Verification items for the finished model (mm, model axes). A direction names the side the tool comes from. Give positions to 0.01 mm unless a question says otherwise; leave off trailing zeros. Loops run counter-clockwise (first coordinate to the right, second up) from the corner with the lowest first, then second, coordinate; pieces in that order, holes last. Notation, with made-up numbers: (-11.75, -8) - (19.25, -8) arc R24 ccw to (19.25, 13) - close; hole circle Ø3 at (-36, 34). An arc over 180 degrees is marked (long way). Answer in a Markdown table with one row per item.
```python
from build123d import *

# Parameters (mm, degrees)
EXTRUDE_1_DEPTH             = 43.4
EXTRUDE_2_DEPTH             = 1.8
CUT_EXTRUDE_1_DEPTH         = 43.4
EXTRUDE_3_DEPTH             = 43.4
EXTRUDE_4_DEPTH             = 16.205128205
SKETCH_6_W                  = 45.2
SKETCH_6_H                  = 41
EXTRUDE_5_DEPTH             = 2
SKETCH_7_W                  = 34
SKETCH_7_H                  = 20
EXTRUDE_6_DEPTH             = 8
EXTRUDE_7_DEPTH             = 1.8
HOLE_WIZARD_3_3_3_3_2_D     = 3.3
HOLE_WIZARD_3_3_3_3_2_DEPTH = 10
HOLE_WIZARD_16_0_16_1_D     = 16
HOLE_WIZARD_16_0_16_1_DEPTH = 55
SKETCH_19_R                 = 1.65
CUT_EXTRUDE_6_DEPTH         = 5


with BuildPart() as part:
    # 草图1 → 凸台-拉伸1 (new body)
    with BuildSketch(Plane(origin=(21.7, 0, 0), x_dir=(0, 0, -1), z_dir=(1, 0, 0))):
        Polygon((-18.205128205, 8), (-18.205128205, 49), (-55, 8), align=None)
    extrude(amount=-EXTRUDE_1_DEPTH)

    # 草图2 → 凸台-拉伸2 (add)
    with BuildSketch(Plane.ZY.offset(21.7)):
        Polygon((18.205128205, 8), (18.205128205, 49), (55, 8), align=None)
    extrude(amount=EXTRUDE_2_DEPTH)

    # 草图3 → 切除-拉伸1 (cut)
    with BuildSketch(Plane(origin=(21.7, 0, 0), x_dir=(0, 0, -1), z_dir=(1, 0, 0))):
        Polygon((-18.205128205, 8), (-18.205128205, 47), (-20, 47), (-55, 8), align=None)
    extrude(amount=-CUT_EXTRUDE_1_DEPTH, mode=Mode.SUBTRACT)

    # 草图4 → 凸台-拉伸3 (add)
    with BuildSketch(Plane(origin=(-21.7, 0, 0), x_dir=(0, 0, -1), z_dir=(1, 0, 0))):
        Polygon((-18.205128205, 10), (-18.205128205, 8), (-55, 8), (-53.205128205, 10), align=None)
    extrude(amount=EXTRUDE_3_DEPTH)

    # 草图5 → 凸台-拉伸4 (add)
    with BuildSketch(Plane(origin=(0, 0, 18.205128205), x_dir=(-1, 0, 0), z_dir=(0, 0, -1))):
        Polygon((21.7, 10), (21.7, 47), (-21.7, 47), (-21.7, 49), (23.5, 49), (23.5, 8), (-21.7, 8), (-21.7, 10), align=None)
    extrude(amount=EXTRUDE_4_DEPTH)

    # 草图6 → 凸台-拉伸5 (add)
    with BuildSketch(Plane(origin=(0, 0, 2), x_dir=(-1, 0, 0), z_dir=(0, 0, -1))):
        with Locations((0.9, 28.5)):
            Rectangle(SKETCH_6_W, SKETCH_6_H)
    extrude(amount=EXTRUDE_5_DEPTH)

    # 草图7 → 凸台-拉伸6 (add)
    with BuildSketch(Plane.XZ.offset(-8)):
        with Locations((0, 10)):
            Rectangle(SKETCH_7_W, SKETCH_7_H)
    extrude(amount=EXTRUDE_6_DEPTH)

    # 草图10 → 凸台-拉伸7 (add)
    with BuildSketch(Plane(origin=(21.7, 0, 0), x_dir=(0, 0, -1), z_dir=(1, 0, 0))):
        Polygon((0, 49), (0, 8), (-55, 8), (-18.205128205, 49), align=None)
    extrude(amount=EXTRUDE_7_DEPTH)

    # Ø3.3 (3.3) 直径孔2
    with Locations(Plane(origin=(0, 0, 0), x_dir=(-1, 0, 0), z_dir=(0, -1, 0))):
        with Locations((13, -5), (13, -14.75698348)):
            hole_wizard_3_3_3_3_2 = Hole(HOLE_WIZARD_3_3_3_3_2_D / 2, depth=HOLE_WIZARD_3_3_3_3_2_DEPTH)

    # Ø16.0 (16) 直径孔1
    with Locations(Plane(origin=(0, 0, 0), x_dir=(-1, 0, 0), z_dir=(0, 0, -1))):
        with Locations((0, 0)):
            Hole(HOLE_WIZARD_16_0_16_1_D / 2, depth=HOLE_WIZARD_16_0_16_1_DEPTH)

    # 草图19 → 切除-拉伸6 (cut)
    # profile 1 of 2: a face of its own
    with BuildSketch(Plane(origin=(0, 10, 0), x_dir=(1, 0, 0), z_dir=(0, 1, 0))):
        Polygon((-9.795706006, -14.75698348), (-11.397853003, -11.98198348), (-14.602146997, -11.98198348), (-16.204293994, -14.75698348), (-14.602146997, -17.53198348), (-11.397853003, -17.53198348), align=None)
        with Locations(Location((-13, -14.75698348, 0), (0, 0, 90))):
            Circle(SKETCH_19_R, mode=Mode.SUBTRACT)
    # profile 2 of 2: a face of its own
    with BuildSketch(Plane(origin=(0, 10, 0), x_dir=(1, 0, 0), z_dir=(0, 1, 0))):
        Polygon((-9.795706006, -5), (-11.397853003, -2.225), (-14.602146997, -2.225), (-16.204293994, -5), (-14.602146997, -7.775), (-11.397853003, -7.775), align=None)
        with Locations(Location((-13, -5, 0), (0, 0, 90))):
            Circle(SKETCH_19_R, mode=Mode.SUBTRACT)
    cut_extrude_6 = extrude(amount=-CUT_EXTRUDE_6_DEPTH, mode=Mode.SUBTRACT)

    # 镜向1: Ø3.3 (3.3) 直径孔2, 切除-拉伸6 across plane
    add(hole_wizard_3_3_3_3_2.mirror(Plane.ZY), mode=Mode.SUBTRACT)
    add(cut_extrude_6.mirror(Plane.ZY), mode=Mode.SUBTRACT)


solid = part.part
```
Q1. Tool access check on faces 5 (the face through (-13.4, 2.5, 6.6)), 6 (the face through (13, 8, 17.532)), 7 (the face through (12, 0, 10)). Record the directions out of +Z, -Z, +X, -X, +Y, -Y that give a thin tool (end or side, any length) a straight path to the whole face; none if there is none.
Completed:
| item | result |
|---|---|
| face 5 | -Y |
| face 6 | none |
| face 7 | +Z, -Z, +X, -X, -Y |
Q2. Thickness scan on line 1 (Z direction, x = 13, y = 3); line 2 (X direction, y = 11, z = 49.5); line 3 (Y direction, x = -9.5, z = 13). Record the ranges inside material, lowest first.
Completed:
| item | result |
|---|---|
| line 1 | 0 to 3.35, 6.65 to 13.11, 16.41 to 20 |
| line 2 | -23.5 to -21.7, 21.7 to 23.5 |
| line 3 | 0 to 10, 47 to 49 |
Q3. Sectioned sample at C-C (z = 21). Record the cut outline in (x, y), and give its area (3 significant figures).
Completed:
| item | result |
|---|---|
| outline | (-23.5, 8) - (23.5, 8) - (23.5, 45.89) - (21.7, 45.89) - (21.7, 10) - (-21.7, 10) - (-21.7, 45.89) - (-23.5, 45.89) - close |
| area | 223 mm^2 |
Q4. Sectioned sample at A-A (x = -13). Record the cut outline in (y, z) (3 decimals), and give its area (3 significant figures).
Completed:
| item | result |
|---|---|
| outline | (0, 0) - (49, 0) - (49, 18.205) - (47, 20) - (47, 2) - (10, 2) - (10, 2.225) - (5, 2.225) - (5, 3.35) - (0, 3.35) - close; (0, 6.65) - (5, 6.65) - (5, 7.775) - (10, 7.775) - (10, 11.982) - (5, 11.982) - (5, 13.107) - (0, 13.107) - close; (0, 16.407) - (5, 16.407) - (5, 17.532) - (10, 17.532) - (10, 53.205) - (8, 55) - (8, 20) - (0, 20) - close |
| area | 292 mm^2 |
Q5. Draft check along Y on faces 1 (the face through (0, 49, 9)), 2 (the face through (10.586, 7.535, 3.632)), 3 (the face through (-13, 8, 2.225)), 4 (the face through (-23.5, 24, 22)). Enter one of: +Y half, -Y half, draft (parallel to the pull), parting line (faces both ways), or undercut.
Completed:
| item | result |
|---|---|
| face 1 | +Y half |
| face 2 | undercut |
| face 3 | undercut |
| face 4 | draft |
Q6. Go/stop test with flat-tipped pins: P1, Ø3.5, axis at x = 12.5, y = 6.5, coming from the +Z side; P2, Ø1.5, axis at x = 9.5, z = 32, coming from the +Y side; P3, Ø23.5, axis at x = 3.5, z = 35, coming from the -Y side. Record where each tip stops, or that it passes through.
Completed:
| item | result |
|---|---|
| P1 | z = 55 |
| P2 | y = 10 |
| P3 | y = 8 |
Q7. Sectioned sample at B-B (y = 27.5). Record the cut outline in (x, z).
Completed:
| item | result |
|---|---|
| outline | (-23.5, 0) - (23.5, 0) - (23.5, 37.5) - (21.7, 37.5) - (21.7, 2) - (-21.7, 2) - (-21.7, 37.5) - (-23.5, 37.5) - close |
Q8. Sectioned sample at D-D (x = -4). Record the cut outline in (y, z), and give its area (3 significant figures).
Completed:
| item | result |
|---|---|
| outline | (6.93, 0) - (49, 0) - (49, 18.21) - (47, 20) - (47, 2) - (10, 2) - (10, 53.21) - (8, 55) - (8, 20) - (6.93, 20) - close |
| area | 242 mm^2 |
